Answer from the drawing. Dimensions are ordinates in mm from the lowest x, y and z of the part. A direction names the side the tool comes from. Give positions to 0.01 mm unless a question says otherwise; leave off trailing zeros. Loops run counter-clockwise (first coordinate to the right, second up) from the corner with the lowest first, then second, coordinate; pieces in that order, holes last. Notation, with made-up numbers: (-1, 79.5) - (57, 79.5) arc R21 cw to (57, 106.5) - close; hole circle Ø6 at (21.5, 44). An arc over 180 degrees is marked (long way). One line per item, written item: value.
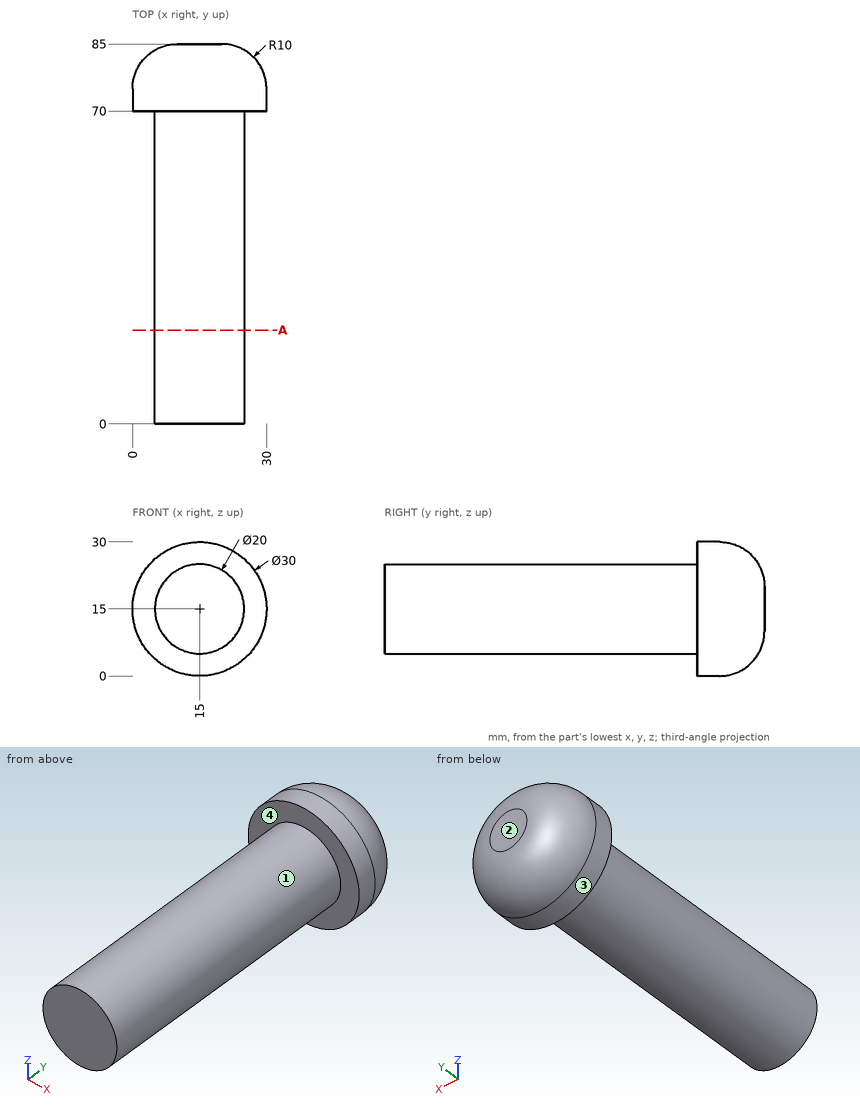
1. The mould has two halves that part along Z. Classify the marked faces 3 and 4: released by +Z, released by -Z, zero draft, split by the parting line, or undercut.
Output:
face 3: split by the parting line
face 4: zero draft
2. Flat-ended cylindrical pins translate along their axes: pin 1 Ø4 at (y, z) = (20.5, 9) entering from -X; pin 2 Ø4 at (y, z) = (31, 5) entering from +X; pin 3 Ø5 at (y, z) = (40, 12.5) entering from +X. Find the tip coordinate at first contact, or state that the pin passes through.
Output:
pin 1: stops at x = 5.83
pin 2: stops at x = 21
pin 3: stops at x = 25
3. Section A-A (y = 21) is taken. Write down the section's boundary in (x, z).
Output:
outline: circle Ø20 at (15, 15)
4. Find the intervals of material crossed by line 1 along Z through (x, y) = (14.5, 16.5); line 2 along Z through (x, y) = (24, 34.5); line 3 along X through (y, z) = (26.5, 16.25), in increasing order.
Output:
line 1: z = 5.01 to 24.99
line 2: z = 10.64 to 19.36
line 3: x = 5.08 to 24.92
5. For the marked faces 1 and 2, determine the directions among +Z, -Z, +X, -X, +Y, -Y from which every point of the face is accessible in a straight line to the end or side of a thin tool.
Output:
face 1: -Y
face 2: +Z, -Z, +X, -X, +Y
